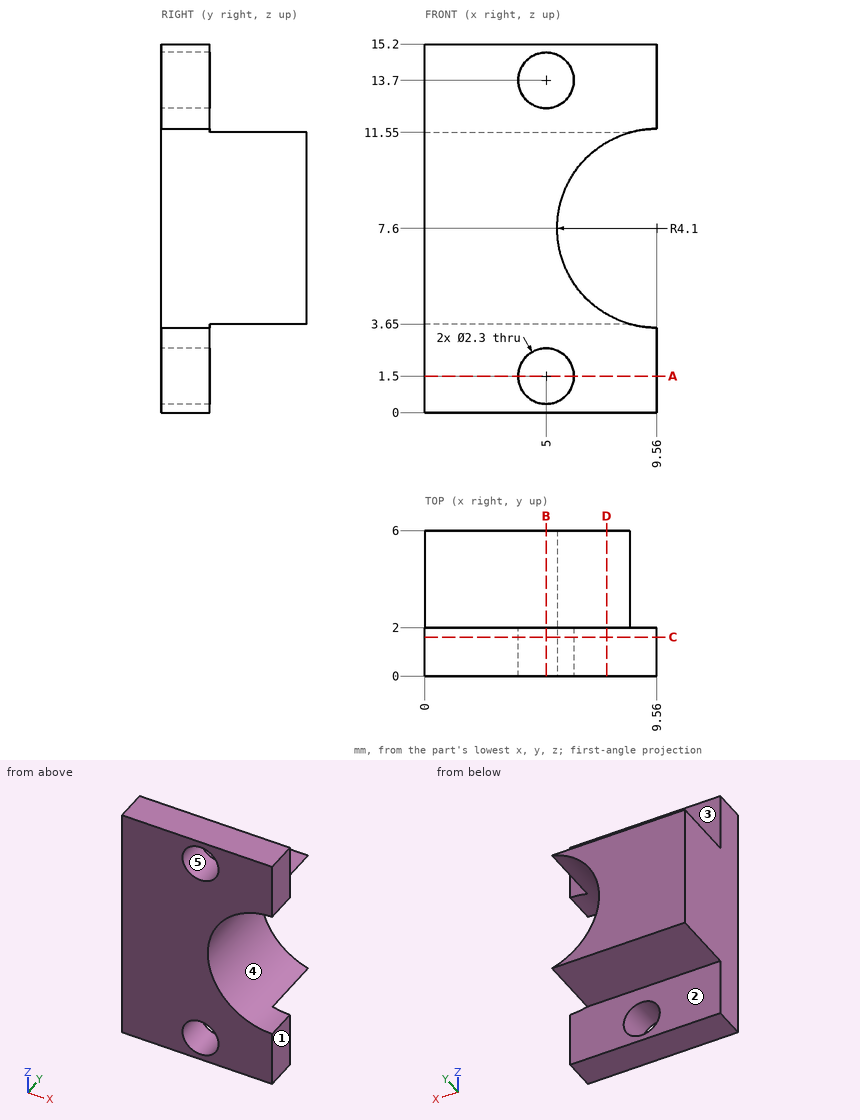
Can you work these out from the drawing? Everything is in mm from the part's minimum corner. A direction names the side the tool comes from. Give positions to 0.01 mm unless a question says otherwise; leave off trailing zeros. Order: outer loops, then holes, each group sorted by start corner. A loop starts at its lowest first (then second) coordinate and runs counter-clockwise, first axis right, second up. Notation, with made-up numbers: M -38,62.25 L -27,62.25 A22 cw -27,75.25 Z; hole C 62,17.5 d3. An arc over 180 degrees is marked long. Use a Markdown table: item, result. Add a question column.
Item 1: Suppose I cut it at A-A (z = 1.5). List the corners of the cut face in (x, y) for me, then the cut area to 3 significant figures.
Item 2: Suppose I cut it at C-C (y = 1.6). List the corners of the cut face in (x, z) for me.
Item 3: Suppose I cut it at B-B (x = 5). List the corners of the cut face in (y, z) for me.
Item 4: Suppose I cut it at D-D (x = 7.5). List the corners of the cut face in (y, z) for me.
Item 5: For the marked faces 1 and 2, which set-ups out of +Z, -Z, +X, -X, +Y, -Y let a thin tool reach every point of the face, with its end or its side?
Item 6: We'd pull the mould along X, two halves only. Please class the marked faces 3, 4 and 5: +X half, -X half, draft (parallel to the pull), parting line (faces both ways), or undercut.
Item 7: If I drill on L1, parallel to Z at x = 5, y = 1.5; L2, parallel to Z at x = 4, y = 1.6; L3, parallel to Z at x = 6, y = 0.7, over which ranges is the centre line in solid material (lowest first)? Write a range as [from, to].
Item 8: Will these pins go through, and if not, where does the flat tip stop? pin 1 (3 mm diameter, centred on x = 3, z = 2, fed in from +Y); pin 2 (2 mm diameter, centred on y = 5, z = 6.5, fed in from +X); pin 3 (3 mm diameter, centred on y = 4.5, z = 9, fed in from +X).
Answer sheet:
| question | item | result |
|---|---|---|
| 1 | outline | M 0,0 L 3.85,0 L 3.85,2 L 0,2 Z; M 6.15,0 L 9.56,0 L 9.56,2 L 6.15,2 Z |
| 1 | area | 14.5 mm² |
| 2 | outline | M 0,0 L 9.56,0 L 9.56,3.5 A4.1 cw 9.56,11.7 L 9.56,15.2 L 0,15.2 Z; hole C 5,1.5 d2.3; hole C 5,13.7 d2.3 |
| 3 | outline | M 0,0 L 2,0 L 2,0.35 L 0,0.35 Z; M 0,2.65 L 2,2.65 L 2,3.65 L 6,3.65 L 6,11.55 L 2,11.55 L 2,12.55 L 0,12.55 Z; M 0,14.85 L 2,14.85 L 2,15.2 L 0,15.2 Z |
| 4 | outline | M 0,0 L 2,0 L 2,3.65 L 6,3.65 L 6,4.06 L 0,4.06 Z; M 0,11.14 L 6,11.14 L 6,11.55 L 2,11.55 L 2,15.2 L 0,15.2 Z |
| 5 | face 1 | +Z, -Z, +X, +Y, -Y |
| 5 | face 2 | -Z, +X, -X, +Y |
| 6 | face 3 | draft |
| 6 | face 4 | +X half |
| 6 | face 5 | undercut |
| 7 | L1 | z = [0, 0.35], [2.65, 12.55], [14.85, 15.2] |
| 7 | L2 | z = [0, 0.93], [2.07, 13.13], [14.27, 15.2] |
| 7 | L3 | z = [0, 0.93], [2.07, 5.57], [9.63, 13.13], [14.27, 15.2] |
| 8 | pin 1 | stops at y = 2 |
| 8 | pin 2 | stops at x = 6.04 |
| 8 | pin 3 | stops at x = 6.66 |
